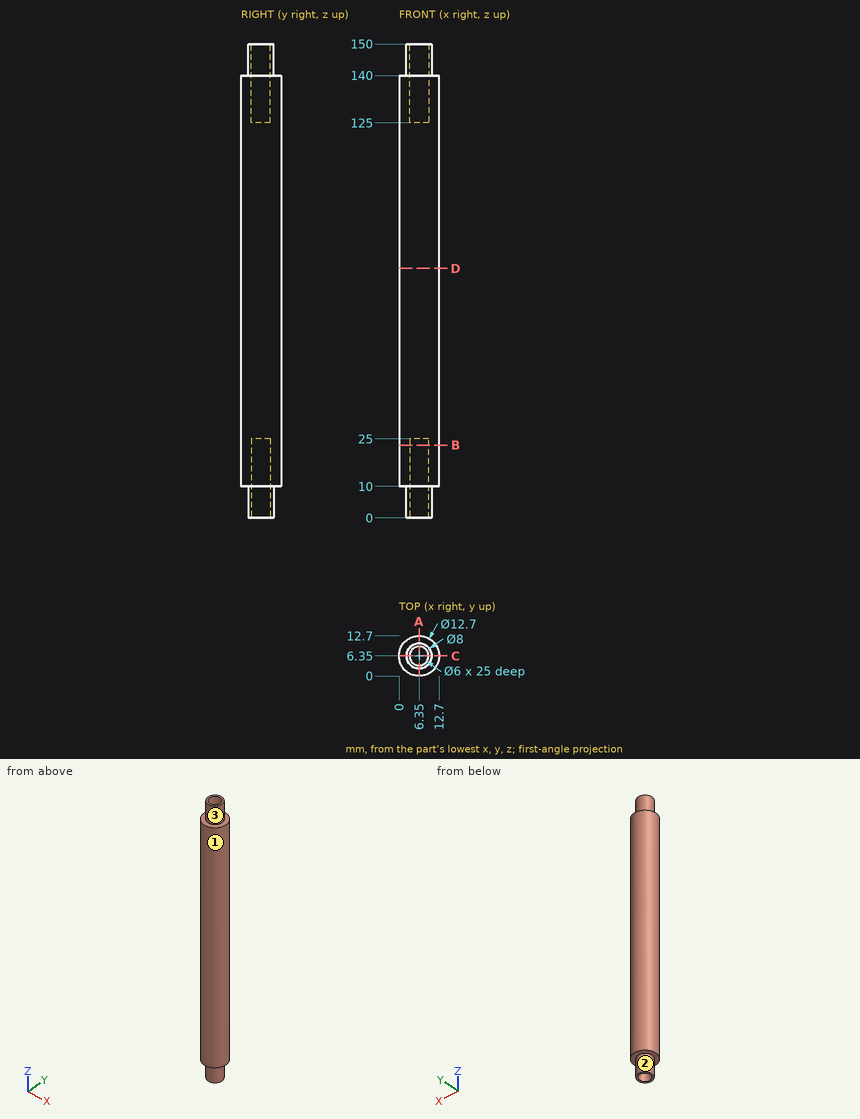
The drawing under review shows one solid part. Ordinate dimensions are in mm from its lowest x, y, z. A direction names the side the tool comes from. Give positions to 0.01 mm unless a question says otherwise; leave off trailing zeros. Loops run counter-clockwise (first coordinate to the right, second up) from the corner with the lowest first, then second, coordinate; pieces in that order, holes last. Notation, with made-up numbers: M 39,-28 L 70,-28 A21 ccw 70,-22 Z; hole C 64.5,50.25 d9. An arc over 180 degrees is marked long. Return JSON: item names as keys, results as strings. Group by question number.
Item 1: Insertion check: pin 1 Ø4 at (x, z) = (3.5, 31.5) entering from +Y. The pin has a flat end and moves straight along its axis. Give the tip position at first contact, or say it passes through.
Item 2: We need section D-D (z = 79). Give the boundary of the cut face in (x, y).
Item 3: We need section A-A (x = 6.35). Give the boundary of the cut face in (y, z), and give its area (3 significant figures).
Item 4: For probe 1 along Y at (x, z) = (6.35, 144.75); probe 2 along Y at (x, z) = (6.35, 131.25); probe 3 along Y at (x, z) = (5.75, 42.5), list the stretches that pass through material, from the lowest coordinate up.
Item 5: We need section B-B (z = 23). Give the boundary of the cut face in (x, y).
Item 6: Tool access review of the marked faces 1, 2 and 3: name each direction out of +Z, -Z, +X, -X, +Y, -Y from which nothing blocks a thin tool from reaching the whole face with its end or side.
Output:
{
 "1": {"pin 1": "stops at y = 12.64"},
 "2": {"outline": "C 6.35,6.35 d12.7"},
 "3": {"outline": "M 0,10 L 2.35,10 L 2.35,0 L 3.35,0 L 3.35,25 L 9.35,25 L 9.35,0 L 10.35,0 L 10.35,10 L 12.7,10 L 12.7,140 L 10.35,140 L 10.35,150 L 9.35,150 L 9.35,125 L 3.35,125 L 3.35,150 L 2.35,150 L 2.35,140 L 0,140 Z", "area": "1,510 mm^2"},
 "4": {"probe 1": "y = 2.35 to 3.35, 9.35 to 10.35", "probe 2": "y = 0 to 3.35, 9.35 to 12.7", "probe 3": "y = 0.03 to 12.67"},
 "5": {"outline": "C 6.35,6.35 d12.7; hole C 6.35,6.35 d6"},
 "6": {"face 1": "+Z, -Z", "face 2": "-Z", "face 3": "+Z"}
}
